Check sheet for the modelled part. Datum: model origin and axes. Units: mm. A direction names the side the tool comes from. Round coordinates to 2 decimals unless told otherwise and drop trailing zeros. Order: outer loops, then holes, each group sorted by start corner. A loop starts at its lowest first (then second) coordinate and runs counter-clockwise, first axis right, second up.
Q1. Depth check by flat-ended pin: P1, Ø12, axis at x = -83.5, y = 26.5, coming from the -Z side; P2, Ø10, axis at x = 37.5, z = -0.5, coming from the -Y side; P3, Ø7, axis at x = -98.57, y = -19.15, coming from the +Z side. Enter the tip coordinate at first touch or a pass-through.
Q2. Cross-section at C-C on z = -4.75. Record the cut outline in (x, y).
Q3. Cross-section at B-B on y = 55. Record the cut outline in (x, z), then the cut area to 3 significant figures.
Q4. Scan lines: probe 1 along X at (y, z) = (-15, 6.5); probe 2 along Z at (x, y) = (-134, -69.5); probe 3 along X at (y, z) = (-9, 7.5). Record each from-to range of solid material in increasing order.
Q5. Set-up check for faces 1 (the cylindrical face through (-150.996, 71.395, -4.437)), 2 (the cylindrical face through (-155.163, -117.902, 6.261)): record each of +Z, -Z, +X, -X, +Y, -Y from which the full face is reachable in a straight line by a thin tool's end or side.
Q6. Cross-section at A-A on x = -96. Record the cut outline in (y, z).
Q7. Mould release check, pull along Y, two halves, no side actions. Record for faces 3 (the flat face through (-44, -18, 6.35)), 4 (the flat face through (-42, -120.753, 6)), 5 (the flat face through (-42, -63, 12.7)): +Y half, -Y half, draft (parallel to the pull), parting line (faces both ways), or undercut.
Q8. Cross-section at D-D on x = 30. Record the cut outline in (y, z).
from build123d import *

# Parameters (mm, degrees)
LID_DEPTH           = 12.7
SKETCH2_R           = 3.25
CORNER_SHAFTS_DEPTH = 9
SKETCH9_R           = 6
WIRE_HOLE_DEPTH     = 201.174580316


with BuildPart() as part:
    # Sketch1 → Lid (new body)
    with BuildSketch(Plane(origin=(-2.566079358, -10, 0), x_dir=(1, 0, 0), z_dir=(0, 0, 1))):
        with BuildLine():
            Line((-145.603603604, 92.446846847), (62.996396396, 92.446846847))
            ThreePointArc((62.996396396, 92.446846847), (70.067464208, 89.517914659), (72.996396396, 82.446846847))
            Line((72.996396396, 82.446846847), (72.996396396, -100.753153153))
            ThreePointArc((72.996396396, -100.753153153), (70.067464208, -107.824220965), (62.996396396, -110.753153153))
            Line((62.996396396, -110.753153153), (-145.603603604, -110.753153153))
            ThreePointArc((-145.603603604, -110.753153153), (-152.674671415, -107.824220965), (-155.603603604, -100.753153153))
            Line((-155.603603604, -100.753153153), (-155.603603604, 82.446846847))
            ThreePointArc((-155.603603604, 82.446846847), (-152.674671415, 89.517914659), (-145.603603604, 92.446846847))
        make_face()
    extrude(amount=LID_DEPTH)

    # Sketch2 → Corner Shafts (add)
    with BuildSketch(Plane.XY):
        with BuildLine():
            Line((60.253540343, -110.576376458), (64.849734421, -115.172570536))
            ThreePointArc((64.849734421, -115.172570536), (64.849734421, -110.576376458), (60.253540343, -110.576376458))
        make_face()
        with Locations((-150.291003305, -112.874473497)):
            Circle(SKETCH2_R)
        with Locations((-150.291003305, 74.56816719)):
            Circle(SKETCH2_R)
        with Locations((62.551637382, 74.56816719)):
            Circle(SKETCH2_R)
    extrude(amount=-CORNER_SHAFTS_DEPTH)

    # Sketch8 → Kinect Loft Cut section 0
    with BuildSketch(Plane.XY.offset(12.7)):
        with BuildLine():
            Line((-8.369682962, 23.346846847), (-79.369682962, 23.346846847))
            Line((-79.369682962, 23.346846847), (-79.369682962, -61.653153153))
            Line((-79.369682962, -61.653153153), (-8.369682962, -61.653153153))
            Line((-8.369682962, -61.653153153), (-8.369682962, 23.346846847))
        make_face()
    # Base for Kinect → Kinect Loft Cut section 1
    with BuildSketch(Plane.XY.offset(6.35)):
        with BuildLine():
            Line((-10.369682962, 21.346846847), (-77.369682962, 21.346846847))
            Line((-77.369682962, 21.346846847), (-77.369682962, -59.653153153))
            Line((-77.369682962, -59.653153153), (-10.369682962, -59.653153153))
            Line((-10.369682962, -59.653153153), (-10.369682962, 21.346846847))
        make_face()
    loft(mode=Mode.SUBTRACT)

    # Sketch9 → Wire Hole (cut, through all)
    with BuildSketch(Plane.XY.offset(12.7)):
        with Locations((-98.566640815, -19.153153153)):
            Circle(SKETCH9_R)
    extrude(amount=-WIRE_HOLE_DEPTH, mode=Mode.SUBTRACT)


solid = part.part
Results found:
1. P1: stops at z = 0
1. P2: stops at y = -120.75
1. P3: passes through
2. outline: circle Ø6.5 at (-150.29, -112.87); circle Ø6.5 at (-150.29, 74.57); circle Ø6.5 at (62.55, 74.57); (60.25, -110.58) - (64.85, -115.17) arc R3.25 ccw to start
3. outline: (-158.17, 0) - (70.43, 0) - (70.43, 12.7) - (-158.17, 12.7) - close
3. area: 2,900 mm2
4. probe 1: x = -158.17 to -102.9, -94.24 to -77.42, -10.32 to 70.43
4. probe 2: z = 0 to 12.7
4. probe 3: x = -158.17 to -77.73, -10.01 to 70.43
5. face 1: -Z
5. face 2: +Z, -Z, -X, -Y
6. outline: (-120.75, 0) - (-24.58, 0) - (-24.58, 12.7) - (-120.75, 12.7) - close; (-13.73, 0) - (82.45, 0) - (82.45, 12.7) - (-13.73, 12.7) - close
7. face 3: undercut
7. face 4: -Y half
7. face 5: draft
8. outline: (-120.75, 0) - (82.45, 0) - (82.45, 12.7) - (-120.75, 12.7) - close
